```python
from build123d import *

# Parameters (mm, degrees)
F6_DEPTH = 2.5


with BuildPart() as f6:
    # F5 (on line) → F6 (new body)
    with BuildSketch(Plane(origin=(0, -22.497566339, -61.8115555092), x_dir=(1, 0, 0), z_dir=(0, 0.3420201433, 0.9396926208))):
        with BuildLine():
            add(Edge.make_bspline(
                [(0, -10.7600335032), (-12.424566783, -10.7759898528), (-25.8446539441, 0.2358042705), (-33.2600735128, 10.1268971339), (-35.0152626634, 23.9554308355)],
                knots=[0, 0, 0, 0, 0.5021229649, 1, 1, 1, 1], degree=3))
            add(Edge.make_bspline(
                [(0, -10.7600335032), (12.424566783, -10.7759898528), (25.8446539441, 0.2358042705), (33.2600735128, 10.1268971339), (35.0152626634, 23.9554308355)],
                knots=[0, 0, 0, 0, 0.5021229649, 1, 1, 1, 1], degree=3))
            Line((35.0152626634, 23.9554308355), (35.0152626634, 82.8513292865))
            Line((35.0152626634, 82.8513292865), (-35.0152626634, 82.8513292865))
            Line((-35.0152626634, 82.8513292865), (-35.0152626634, 23.9554308355))
        make_face()
    extrude(amount=F6_DEPTH)


solid = f6.part
```
Source: CAD feature listing. Evaluate the final solid. Frame: model axes, mm. Give positions to 0.01 mm unless a question says otherwise; leave off trailing zeros. Loops run counter-clockwise (first coordinate to the right, second up) from the corner with the lowest first, then second, coordinate; pieces in that order, holes last. Notation, with made-up numbers: (25, 59.5) -> (45, 59.5) arc R17 cw to (45, 65.5) -> close; hole circle Ø11 at (28, -23). An arc over 180 degrees is marked (long way). Put each result on its own line as item: value. Start each with the question number.
1) Cut plane A-A (y = 36.5). Return loops of the section in (x, z).
2) Contact query for flat-ended pins moving along their axis: P1, Ø6, axis at x = 4.5, y = 33, coming from the -Z side; P2, Ø1, axis at x = 22, y = 43.5, coming from the +Z side; P3, Ø8, axis at x = -14, y = 7.5, coming from the +Z side; P4, Ø12, axis at y = 32, z = -78.5, coming from the +X side. Output: stop coordinate, or through.
3) Material intervals for probe 1 along Z at (x, y) = (12, 48); probe 2 along Z at (x, y) = (-30.5, 2.5); probe 3 along X at (y, z) = (-26, -59.5), sorted ascending.
4) Cut plane B-B (z = -79). Return loops of the section in (x, y).
Results are:
1. outline: (-35.02, -83.28) -> (35.02, -83.28) -> (35.02, -80.62) -> (-35.02, -80.62) -> close
2. P1: stops at z = -83.1
2. P2: stops at z = -82.99
2. P3: stops at z = -68.61
2. P4: stops at x = 35.02
3. probe 1: z = -87.47 to -84.81
3. probe 2: z = -70.91 to -68.25
3. probe 3: x = -19.89 to 19.89
4. outline: (-35.02, 24.73) -> (35.02, 24.73) -> (35.02, 32.04) -> (-35.02, 32.04) -> close
